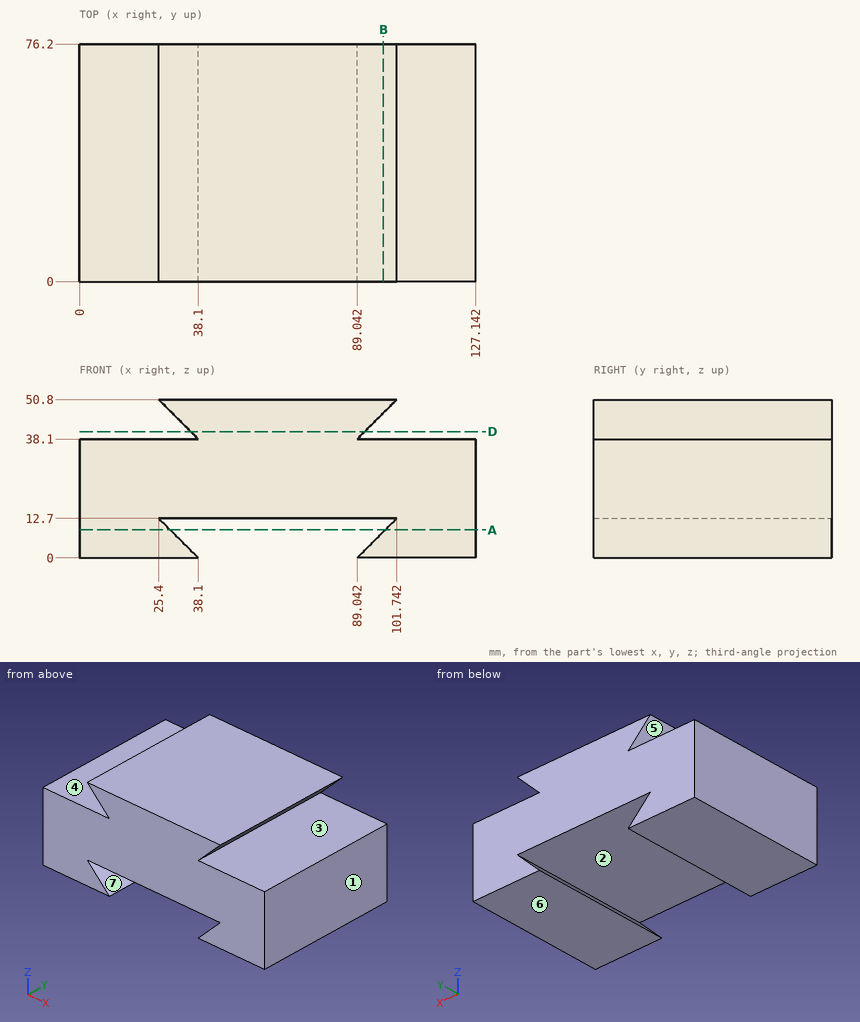
Check sheet for the drawn part. Datum: minimum x, y, z corner. Units: mm. A direction names the side the tool comes from. Give positions to 0.01 mm unless a question says otherwise; leave off trailing zeros. Order: outer loops, then holes, each group sorted by start corner. A loop starts at its lowest first (then second) coordinate and runs counter-clockwise, first axis right, second up. Notation, with made-up numbers: (-35.75, -27) - (-3.75, -27) arc R32 cw to (-3.75, 6) - close; hole circle Ø6 at (-6.5, 83). An arc over 180 degrees is marked (long way). Write item = value, one per line. Start each with the question number.
1) Scan lines: L1, parallel to Z at x = 27.5, y = 72; L2, parallel to Z at x = 37.5, y = 3; L3, parallel to Z at x = 60, y = 34.5. Record each from-to range of solid material in increasing order.
2) Section check A-A (z = 9). Enter the section's corners in (x, y).
3) Section check D-D (z = 40.5). Enter the section's corners in (x, y).
4) Draft check along X on the marked faces 5, 6 and 7. Enter one of: released by +X, released by -X, zero draft, split by the parting line, or undercut.
5) Gauge pin test, flat ends, axial feed: pin 1 Ø10 at (x, y) = (51, 44) entering from -Z; pin 2 Ø19 at (x, y) = (114.5, 23) entering from +Z. Record the tip position at first contact, or that the pin passes through.
6) Access from +Z, -Z, +X, -X, +Y, -Y to the whole of each face (thin tool, end or side, straight path). Record for the marked faces 1, 2, 3 and 4.
7) Section check B-B (x = 97.5). Enter the section's corners in (y, z).
Geometry check:
q1.L1 = 0 to 10.6, 12.7 to 38.1, 48.7 to 50.8
q1.L2 = 0 to 0.6, 12.7 to 38.1, 38.7 to 50.8
q1.L3 = 12.7 to 50.8
q2.outline = (0, 0) - (29.1, 0) - (29.1, 76.2) - (0, 76.2) - close; (98.04, 0) - (127.14, 0) - (127.14, 76.2) - (98.04, 76.2) - close
q3.outline = (35.7, 0) - (91.44, 0) - (91.44, 76.2) - (35.7, 76.2) - close
q4.face_5 = released by -X
q4.face_6 = zero draft
q4.face_7 = undercut
q5.pin_1 = 12.7
q5.pin_2 = 38.1
q6.face_1 = +Z, -Z, +X, +Y, -Y
q6.face_2 = +Y, -Y
q6.face_3 = +X, +Y, -Y
q6.face_4 = -X, +Y, -Y
q7.outline = (0, 0) - (76.2, 0) - (76.2, 8.46) - (0, 8.46) - close; (0, 12.7) - (76.2, 12.7) - (76.2, 38.1) - (0, 38.1) - close; (0, 46.56) - (76.2, 46.56) - (76.2, 50.8) - (0, 50.8) - close
